Part model, mm, in its own coordinate system. Face numbers are marked on the shaded views. Give positions to 0.01 mm unless a question says otherwise; leave off trailing zeros. Loops run counter-clockwise (first coordinate to the right, second up) from the corner with the lowest first, then second, coordinate; pieces in that order, holes last. Notation, with made-up numbers: M 19.5,-14 L 73.5,-14 A29 cw 73.5,6 Z; hole C -34,68.25 d2. An arc over 180 degrees is marked long. Answer in a Markdown table with one row per item.
from build123d import *

# Parameters (mm, degrees)
BOSS_EXTRU_1_DEPTH = 191


with BuildPart() as part:
    # Esquisse1 → Boss.-Extru.1 (new body)
    with BuildSketch(Plane.XY):
        with BuildLine():
            Line((-39.529333289, 16.90370196), (-39.335219005, 16.17925759))
            ThreePointArc((-39.335219005, 16.17925759), (-18.25, 0), (-39.335219005, -16.17925759))
            Line((-39.335219005, -16.17925759), (-39.529333289, -16.90370196))
            ThreePointArc((-39.529333289, -16.90370196), (-37.17213026, -18.592337614), (-34.635254916, -19.996673749))
            ThreePointArc((-34.635254916, -19.996673749), (-34.68750182, -22.895840311), (-34.40370196, -25.781555843))
            Line((-34.40370196, -25.781555843), (-33.67925759, -25.975670127))
            ThreePointArc((-33.67925759, -25.975670127), (-9.125, -15.804963619), (-5.655961415, -42.154927717))
            Line((-5.655961415, -42.154927717), (-5.125631329, -42.685257803))
            ThreePointArc((-5.125631329, -42.685257803), (-2.48462844, -41.488177925), (0, -39.993347498))
            ThreePointArc((0, -39.993347498), (2.48462844, -41.488177925), (5.125631329, -42.685257803))
            Line((5.125631329, -42.685257803), (5.655961415, -42.154927717))
            ThreePointArc((5.655961415, -42.154927717), (9.125, -15.804963619), (33.67925759, -25.975670127))
            Line((33.67925759, -25.975670127), (34.40370196, -25.781555843))
            ThreePointArc((34.40370196, -25.781555843), (34.68750182, -22.895840311), (34.635254916, -19.996673749))
            ThreePointArc((34.635254916, -19.996673749), (37.17213026, -18.592337614), (39.529333289, -16.90370196))
            Line((39.529333289, -16.90370196), (39.335219005, -16.17925759))
            ThreePointArc((39.335219005, -16.17925759), (18.25, 0), (39.335219005, 16.17925759))
            Line((39.335219005, 16.17925759), (39.529333289, 16.90370196))
            ThreePointArc((39.529333289, 16.90370196), (37.17213026, 18.592337614), (34.635254916, 19.996673749))
            ThreePointArc((34.635254916, 19.996673749), (34.68750182, 22.895840311), (34.40370196, 25.781555843))
            Line((34.40370196, 25.781555843), (33.67925759, 25.975670127))
            ThreePointArc((33.67925759, 25.975670127), (9.125, 15.804963619), (5.655961415, 42.154927717))
            Line((5.655961415, 42.154927717), (5.125631329, 42.685257803))
            ThreePointArc((5.125631329, 42.685257803), (2.48462844, 41.488177925), (0, 39.993347498))
            ThreePointArc((0, 39.993347498), (-2.48462844, 41.488177925), (-5.125631329, 42.685257803))
            Line((-5.125631329, 42.685257803), (-5.655961415, 42.154927717))
            ThreePointArc((-5.655961415, 42.154927717), (-9.125, 15.804963619), (-33.67925759, 25.975670127))
            Line((-33.67925759, 25.975670127), (-34.40370196, 25.781555843))
            ThreePointArc((-34.40370196, 25.781555843), (-34.68750182, 22.895840311), (-34.635254916, 19.996673749))
            ThreePointArc((-34.635254916, 19.996673749), (-37.17213026, 18.592337614), (-39.529333289, 16.90370196))
        make_face()
    extrude(amount=BOSS_EXTRU_1_DEPTH)


solid = part.part
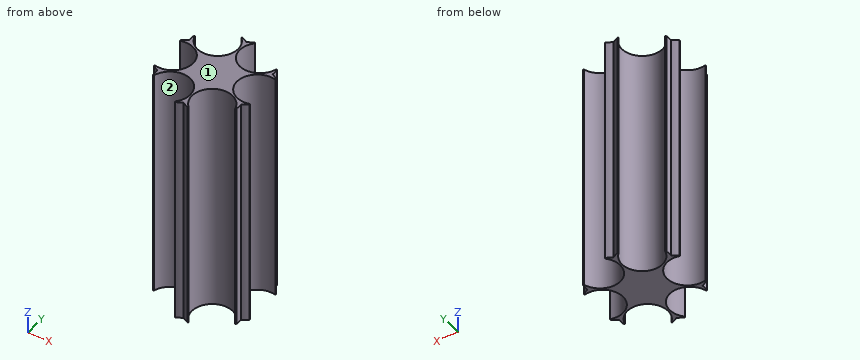
(1) Saw through at C-C (x = 23). Write the cut outline in (y, z).
Recorded:
| item | result |
|---|---|
| outline | M -14.49,0 L -11.69,0 L -11.69,191 L -14.49,191 Z; M 11.69,0 L 14.49,0 L 14.49,191 L 11.69,191 Z |
(2) Saw through at A-A (x = 31). Write the cut outline in (y, z).
Recorded:
| item | result |
|---|---|
| outline | M -20.4,0 L -16.27,0 L -16.27,191 L -20.4,191 Z; M 16.27,0 L 20.4,0 L 20.4,191 L 16.27,191 Z |
(3) Saw through at D-D (y = 0). Write the cut outline in (x, z), plus the area to 3 significant figures.
Recorded:
| item | result |
|---|---|
| outline | M -18.25,0 L 18.25,0 L 18.25,191 L -18.25,191 Z |
| area | 6,970 mm^2 |
(4) Pin check, flat tips, straight feed: pin 1 Ø4 at (y, z) = (4.5, 19) entering from -X; pin 2 Ø3 at (y, z) = (14, 78.5) entering from +X; pin 3 Ø12 at (y, z) = (30.5, 50.5) entering from -X; pin 4 Ø12 at (x, y) = (23.5, -30) entering from +Z. Stop position of each tip, or through.
Recorded:
| item | result |
|---|---|
| pin 1 | stops at x = -19.56 |
| pin 2 | stops at x = 28.65 |
| pin 3 | stops at x = -34.57 |
| pin 4 | passes through |
(5) Drill centre lines: line 1 along X through (y, z) = (17.5, 89); line 2 along X through (y, z) = (-21, 135.5); line 3 along Y through (x, z) = (17.5, 97.5). Where is each one in solid material? Low to high.
Recorded:
| item | result |
|---|---|
| line 1 | x = -38.76 to -28.29, -6.71 to 6.71, 28.29 to 38.76 |
| line 2 | x = -34.69 to -31.42, -3.58 to 3.58, 31.42 to 34.69 |
| line 3 | y = -13.56 to 13.56 |
(6) Pull direction Y, two halves, no side cores. Call the marked faces 1 and 2: +Y half, -Y half, draft (parallel to the pull), parting line (faces both ways), or undercut.
Recorded:
| item | result |
|---|---|
| face 1 | draft |
| face 2 | undercut |
